Read the model definition and answer for the solid it produces. Units are mm, in the model's axes. Face numbers are marked on the shaded views. A direction names the side the tool comes from. Coordinates: 2 decimals unless noted, no trailing zeros. Write each loop counter-clockwise with the first axis right and the second up, starting at its lowest first coordinate (ties: lowest second). Pieces come first, ordered by that corner, then holes. Notation, with made-up numbers: (47, -31.75) -> (88, -31.75) arc R13 ccw to (88, -7.75) -> close; hole circle Ø9 at (24.25, -1). An arc over 180 degrees is marked (long way). Use CSV: the item, a comma, the result in double quotes. Start each with the question number.
from build123d import *

# Parameters (mm, degrees)
SKETCH1_W                      = 33
SKETCH1_H                      = 39.4
BOSS_EXTRUDE1_DEPTH            = 6.35
CBORE_FOR_M3_SHCS1_D           = 3.4
CBORE_FOR_M3_SHCS1_CBORE_D     = 6.5
CBORE_FOR_M3_SHCS1_CBORE_DEPTH = 3
M4_CLEARANCE_HOLE1_D           = 4.5
FILLET1_R                      = 2


with BuildPart() as part:
    # Sketch1 → Boss-Extrude1 (new body)
    with BuildSketch(Plane.XY):
        Rectangle(SKETCH1_W, SKETCH1_H)
    extrude(amount=BOSS_EXTRUDE1_DEPTH)

    # CBORE for M3 SHCS1 (through all)
    with Locations(Plane.XY.offset(6.35)):
        with Locations((-10, 0), (0, 0), (10, 0)):
            CounterBoreHole(CBORE_FOR_M3_SHCS1_D / 2, CBORE_FOR_M3_SHCS1_CBORE_D / 2, CBORE_FOR_M3_SHCS1_CBORE_DEPTH)

    # M4 Clearance Hole1 (through all)
    with Locations(Plane.XY.offset(6.35)):
        with Locations((-13, 13), (-13, -13), (13, -13), (13, 13)):
            Hole(M4_CLEARANCE_HOLE1_D / 2)

    # Fillet1
    fillet1_edges = [part.edges().sort_by_distance(p)[0] for p in [
        (-16.5, 19.7, 3.175),
        (16.5, 19.7, 3.175),
        (16.5, -19.7, 3.175),
        (-16.5, -19.7, 3.175),
    ]]
    fillet(fillet1_edges, radius=FILLET1_R)


solid = part.part
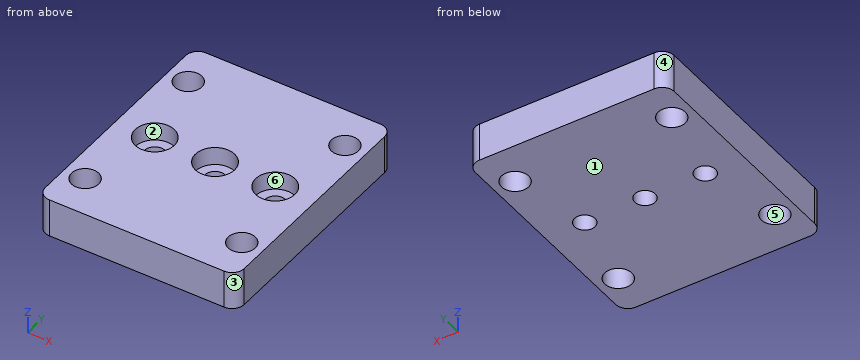
1) Each of these flat-tipped pins is pushed along its axis until it touches: pin 1 (2.5 mm diameter, centred on x = 10, y = 0, fed in from -Z); pin 2 (3 mm diameter, centred on x = 0, y = 0.5, fed in from +Z); pin 3 (12 mm diameter, centred on x = -13, y = 7.5, fed in from -Z). Where does it stop, or does it pass through?
2) The mould has two halves that part along X. Classify the marked faces 3, 4, 5 and 6: pulls with the +X half, pulls with the -X half, needs draft (parallel to the pull), parting line crosses it, or undercut.
3) Section D-D, the plane y = 0 is taken. Give the vertices of the cut face in (x, z).
4) Section C-C, the plane z = 1 is taken. Give the vertices of the cut face in (x, y), plus the area to 3 significant figures.
5) Section A-A, the plane y = -13 is taken. Give the vertices of the cut face in (x, z).
6) Which of the six approach directions +Z, -Z, +X, -X, +Y, -Y give full straight-line access (tool end or side, diameter ignored) to the marked faces 1 and 2?
7) Section B-B, the plane x = 0 is taken. Give the vertices of the cut face in (y, z).
8) Find the intervals of material crossed by line 1 along Y through (x, z) = (-13, 2.25); line 2 along X through (y, z) = (-11, 4.25); line 3 along X through (y, z) = (0.5, 1.25), in increasing order.
The answers:
1,pin 1,"passes through"
1,pin 2,"stops at z = 3.35"
1,pin 3,"stops at z = 0"
2,face 3,"pulls with the +X half"
2,face 4,"pulls with the -X half"
2,face 5,"undercut"
2,face 6,"undercut"
3,outline,"(-16.5, 0) -> (-11.7, 0) -> (-11.7, 3.35) -> (-13.25, 3.35) -> (-13.25, 6.35) -> (-16.5, 6.35) -> close; (-8.3, 0) -> (-1.7, 0) -> (-1.7, 3.35) -> (-3.25, 3.35) -> (-3.25, 6.35) -> (-6.75, 6.35) -> (-6.75, 3.35) -> (-8.3, 3.35) -> close; (1.7, 0) -> (8.3, 0) -> (8.3, 3.35) -> (6.75, 3.35) -> (6.75, 6.35) -> (3.25, 6.35) -> (3.25, 3.35) -> (1.7, 3.35) -> close; (11.7, 0) -> (16.5, 0) -> (16.5, 6.35) -> (13.25, 6.35) -> (13.25, 3.35) -> (11.7, 3.35) -> close"
4,outline,"(-16.5, -17.7) arc R2 ccw to (-14.5, -19.7) -> (14.5, -19.7) arc R2 ccw to (16.5, -17.7) -> (16.5, 17.7) arc R2 ccw to (14.5, 19.7) -> (-14.5, 19.7) arc R2 ccw to (-16.5, 17.7) -> close; hole circle Ø4.5 at (-13, -13); hole circle Ø4.5 at (-13, 13); hole circle Ø3.4 at (-10, 0); hole circle Ø3.4 at (0, 0); hole circle Ø3.4 at (10, 0); hole circle Ø4.5 at (13, -13); hole circle Ø4.5 at (13, 13)"
4,area,"1,210 mm^2"
5,outline,"(-16.5, 0) -> (-15.25, 0) -> (-15.25, 6.35) -> (-16.5, 6.35) -> close; (-10.75, 0) -> (10.75, 0) -> (10.75, 6.35) -> (-10.75, 6.35) -> close; (15.25, 0) -> (16.5, 0) -> (16.5, 6.35) -> (15.25, 6.35) -> close"
6,face 1,"-Z, +X, -X, +Y, -Y"
6,face 2,"+Z"
7,outline,"(-19.7, 0) -> (-1.7, 0) -> (-1.7, 3.35) -> (-3.25, 3.35) -> (-3.25, 6.35) -> (-19.7, 6.35) -> close; (1.7, 0) -> (19.7, 0) -> (19.7, 6.35) -> (3.25, 6.35) -> (3.25, 3.35) -> (1.7, 3.35) -> close"
8,line 1,"y = -19.7 to -15.25, -10.75 to 10.75, 15.25 to 19.7"
8,line 2,"x = -16.5 to -14.03, -11.97 to 11.97, 14.03 to 16.5"
8,line 3,"x = -16.5 to -11.62, -8.38 to -1.62, 1.62 to 8.38, 11.62 to 16.5"
